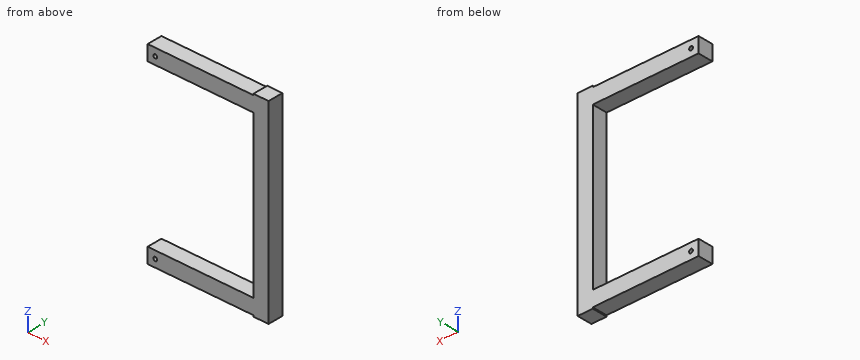
```python
from build123d import *

# Parameters (mm, degrees)
F0_W      = 457.2
F0_H      = 76.2
F1_DEPTH  = 76.2
F2_DEPTH  = 152.4
F3_W      = 76.2
F3_H      = 76.2
F4_DEPTH  = 895.35
F5_W      = 76.2
F5_H      = 76.2
F12_DEPTH = 6.35
F6_W      = 76.2
F6_H      = 76.2
F7_DEPTH  = 533.4
F9_DEPTH  = 76.2
F11_DEPTH = 76.2


with BuildPart() as f1:
    # F0 (on Top) → F1 (new body)
    with BuildSketch(Plane.XY):
        with Locations((4.4659457539, 3.0175000429)):
            Rectangle(F0_W, F0_H)
    extrude(amount=F1_DEPTH)

    # F2 (add): a face of the model
    f2_faces = [f1.faces().sort_by_distance(p)[0] for p in [
        (233.0659457539, 3.0175000429, 38.1),
    ]]
    extrude(f2_faces, amount=F2_DEPTH)

    # F3 (on face) → F4 (join)
    with BuildSketch(Plane.XY.offset(76.2)):
        with Locations((347.3659457539, 3.0175000429)):
            Rectangle(F3_W, F3_H)
    extrude(amount=F4_DEPTH)

    # F5 (on face) → F12 (join)
    with BuildSketch(Plane(origin=(0, 0, 0), x_dir=(1, 0, 0), z_dir=(0, 0, -1))):
        with Locations((347.3659457539, -3.0175000429)):
            Rectangle(F5_W, F5_H)
    extrude(amount=F12_DEPTH)

    # F6 (on face) → F7 (join)
    with BuildSketch(Plane(origin=(309.2659457539, 0, 0), x_dir=(0, -1, 0), z_dir=(-1, 0, 0))):
        with Locations((-3.0175000429, 927.1)):
            Rectangle(F6_W, F6_H)
    extrude(amount=F7_DEPTH)

    # F8 (on face) → F9 (cut)
    with BuildSketch(Plane.XZ.offset(35.0824999571)):
        with BuildLine():
            ThreePointArc((-195.5590542461, 927.1), (-186.0340542461, 917.575), (-176.5090542461, 927.1))
            ThreePointArc((-176.5090542461, 927.1), (-186.0340542461, 936.625), (-195.5590542461, 927.1))
        make_face()
    extrude(amount=-F9_DEPTH, mode=Mode.SUBTRACT)

    # F10 (on face) → F11 (cut)
    with BuildSketch(Plane.XZ.offset(35.0824999571)):
        with BuildLine():
            ThreePointArc((-176.5090542461, 38.1), (-186.0340542461, 47.625), (-195.5590542461, 38.1))
            ThreePointArc((-195.5590542461, 38.1), (-186.0340542461, 28.575), (-176.5090542461, 38.1))
        make_face()
    extrude(amount=-F11_DEPTH, mode=Mode.SUBTRACT)


solid = f1.part
```
CAD build for the part. Positions are in the model's coordinates, mm. Round coordinates to 2 decimals unless told otherwise and drop trailing zeros. Order: outer loops, then holes, each group sorted by start corner. A loop starts at its lowest first (then second) coordinate and runs counter-clockwise, first axis right, second up.
Q1. Slice it at B-B (y = 15). Write the cut outline in (x, z) (3 decimals), and give its area (3 significant figures).
Q2. Wall check: L1, parallel to Z at x = -14, y = -7; L2, parallel to X at y = -17, z = 927.1; L3, parallel to X at y = -8.5, z = 697. Give the ranges that are in metal, low to high.
Q3. Drop flat-ended pins along their axis: pin 1 (1.9 mm diameter, centred on y = 8, z = -2, fed in from -X); pin 2 (1 mm diameter, centred on x = 76, y = 5.5, fed in from +Z); pin 3 (2 mm diameter, centred on x = 280.5, y = 2, fed in from -Z). Give the stop position or say it passes through.
Q4. Slice it at D-D (z = 422). Write the cut outline in (x, y).
Q5. Slice it at C-C (x = 78). Write the cut outline in (y, z), and give its area (3 significant figures).
Q6. Slice it at A-A (z = 927.1). Write the cut outline in (x, y), and give its area (3 significant figures).
Results below:
1. outline: (-224.134, 0) - (309.266, 0) - (309.266, -6.35) - (385.466, -6.35) - (385.466, 971.55) - (309.266, 971.55) - (309.266, 965.2) - (-224.134, 965.2) - (-224.134, 889) - (309.266, 889) - (309.266, 76.2) - (-224.134, 76.2) - close; hole circle Ø19.05 at (-186.034, 38.1); hole circle Ø19.05 at (-186.034, 927.1)
1. area: 155,000 mm2
2. L1: z = 0 to 76.2, 889 to 965.2
2. L2: x = -224.13 to -195.56, -176.51 to 385.47
2. L3: x = 309.27 to 385.47
3. pin 1: stops at x = 309.27
3. pin 2: stops at z = 965.2
3. pin 3: stops at z = 0
4. outline: (309.27, -35.08) - (385.47, -35.08) - (385.47, 41.12) - (309.27, 41.12) - close
5. outline: (-35.08, 0) - (41.12, 0) - (41.12, 76.2) - (-35.08, 76.2) - close; (-35.08, 889) - (41.12, 889) - (41.12, 965.2) - (-35.08, 965.2) - close
5. area: 11,600 mm2
6. outline: (-224.13, -35.08) - (-195.56, -35.08) - (-195.56, 41.12) - (-224.13, 41.12) - close; (-176.51, -35.08) - (385.47, -35.08) - (385.47, 41.12) - (-176.51, 41.12) - close
6. area: 45,000 mm2
